Verification items for the finished model (mm, model axes). Face numbers are marked on the shaded views. A direction names the side the tool comes from. Round coordinates to 2 decimals unless told otherwise and drop trailing zeros. Write each loop counter-clockwise with the first axis right and the second up, starting at its lowest first coordinate (ties: lowest second). Pieces come first, ordered by that corner, then holes. Notation, with made-up numbers: (-35.75, -21) - (-14.75, -21) arc R27 cw to (-14.75, 0) - close; hole circle Ø6 at (-21.5, -11). An arc over 180 degrees is marked (long way). Answer as a JSON object with one key per item and string values. Group by question number.
1) Go/stop test with flat-tipped pins: pin 1 Ø3 at (y, z) = (-12, 8.5) entering from +X; pin 2 Ø7.5 at (y, z) = (-29, 6) entering from -X; pin 3 Ø2.5 at (x, z) = (42.5, 4.5) entering from +Y. Record where each tip stops, or that it passes through.
2) Section check A-A (y = -4). Enter the section's corners in (x, z), then the cut area to 4 significant figures.
3) Thickness scan on line 1 (Y direction, x = 10.5, z = 3); line 2 (X direction, y = 10, z = 6.75); line 3 (X direction, y = -0.5, z = 8). Record the ranges inside material, lowest first.
4) Mould release check, pull along X, two halves, no side actions. Record for the marked faces 4, 5 and 6: +X half, -X half, draft (parallel to the pull), parting line (faces both ways), or undercut.
5) Section check D-D (x = -37.5). Enter the section's corners in (y, z), then the cut area to 4 significant figures.
6) Section check C-C (z = 6.75). Enter the section's corners in (x, y).
7) Set-up check for the marked faces 1, 2 and 3: record each of +Z, -Z, +X, -X, +Y, -Y from which the full face is reachable in a straight line by a thin tool's end or side.
8) Section check B-B (x = -24). Enter the section's corners in (y, z).
```python
from build123d import *

# Parameters (mm, degrees)
SKETCH_1_W          = 5
SKETCH_1_H          = 10
SKETCH_1_W_2        = 100.5
SKETCH_1_H_2        = 80.5
SKETCH_1_W_3        = 6
SKETCH_1_H_3        = 7.5
SKETCH_1_W_4        = 53
SKETCH_1_H_4        = 53
EXTRUDE_1_DEPTH     = 15
SKETCH_2_W          = 59
SKETCH_2_H          = 59
CUT_EXTRUDE_1_DEPTH = 10


with BuildPart() as part:
    # 草圖1 → 填料-伸長1 (new body)
    with BuildSketch(Plane.XY):
        with Locations((-62.305536773, -5.054)):
            Rectangle(SKETCH_1_W, SKETCH_1_H)
        with Locations((-9.555536773, -5.304)):
            Rectangle(SKETCH_1_W_2, SKETCH_1_H_2)
        with Locations((30.944463227, -28.304)):
            Rectangle(SKETCH_1_W_3, SKETCH_1_H_3, mode=Mode.SUBTRACT)
        with Locations((-9.555536773, 0.446)):
            Rectangle(SKETCH_1_W_4, SKETCH_1_H_4, mode=Mode.SUBTRACT)
        with Locations((43.194463227, -5.054)):
            Rectangle(SKETCH_1_W, SKETCH_1_H)
    extrude(amount=EXTRUDE_1_DEPTH)

    # 草圖2 → 除料-伸長1 (cut)
    with BuildSketch(Plane.XY.offset(15)):
        with Locations((-9.555536773, 0.446)):
            Rectangle(SKETCH_2_W, SKETCH_2_H)
    extrude(amount=-CUT_EXTRUDE_1_DEPTH, mode=Mode.SUBTRACT)


solid = part.part
```
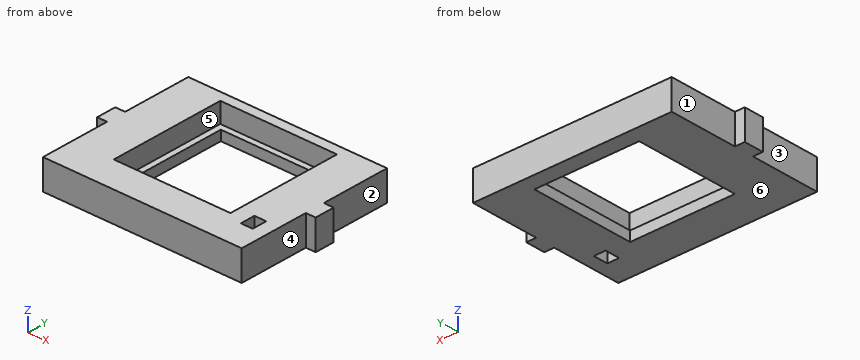
Returned:
{
 "1": {"pin 1": "x = 40.69", "pin 2": "x = -59.81", "pin 3": "y = -0.05"},
 "2": {"outline": "(-64.81, 0) - (-36.06, 0) - (-36.06, 5) - (-39.06, 5) - (-39.06, 15) - (-64.81, 15) - close; (16.94, 0) - (45.69, 0) - (45.69, 15) - (19.94, 15) - (19.94, 5) - (16.94, 5) - close", "area": "802.5 mm2"},
 "3": {"line 1": "-45.55 to -26.05, 26.95 to 34.95", "line 2": "-59.81 to -39.06, 19.94 to 40.69", "line 3": "-64.81 to -39.06, 19.94 to 45.69"},
 "4": {"face 4": "+X half", "face 5": "undercut", "face 6": "draft"},
 "5": {"outline": "(-45.55, 0) - (34.95, 0) - (34.95, 15) - (29.95, 15) - (29.95, 5) - (-29.05, 5) - (-29.05, 15) - (-45.55, 15) - close", "area": "617.5 mm2"},
 "6": {"outline": "(-64.81, -10.05) - (-59.81, -10.05) - (-59.81, -45.55) - (40.69, -45.55) - (40.69, -10.05) - (45.69, -10.05) - (45.69, -0.05) - (40.69, -0.05) - (40.69, 34.95) - (-59.81, 34.95) - (-59.81, -0.05) - (-64.81, -0.05) - close; hole (-39.06, -29.05) - (19.94, -29.05) - (19.94, 29.95) - (-39.06, 29.95) - close; hole (27.94, -32.05) - (33.94, -32.05) - (33.94, -24.55) - (27.94, -24.55) - close"},
 "7": {"face 1": "+Z, -Z, -X, +Y", "face 2": "+Z, -Z, +X, +Y", "face 3": "+Z, -Z, -X, -Y"},
 "8": {"outline": "(-45.55, 0) - (-26.05, 0) - (-26.05, 5) - (-29.05, 5) - (-29.05, 15) - (-45.55, 15) - close; (26.95, 0) - (34.95, 0) - (34.95, 15) - (29.95, 15) - (29.95, 5) - (26.95, 5) - close"}
}
